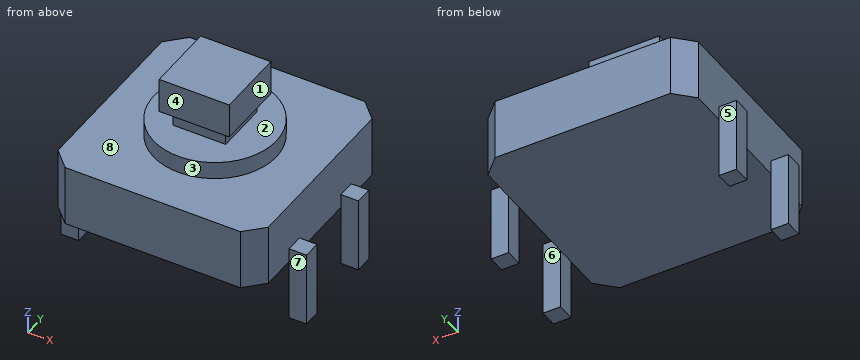
```python
from build123d import *

# Parameters (mm, degrees)
SKETCH_1_W      = 12
SKETCH_1_H      = 12
EXTRUDE_1_DEPTH = 3.5
SKETCH_2_R      = 3.5
EXTRUDE_2_DEPTH = 1
SKETCH_3_W      = 3
SKETCH_3_H      = 3
EXTRUDE_3_DEPTH = 1
SKETCH_4_W      = 4
SKETCH_4_H      = 4
EXTRUDE_4_DEPTH = 2
SKETCH_5_W      = 4.3
SKETCH_5_H      = 1
EXTRUDE_5_DEPTH = 1
SKETCH_7_W      = 4.3
SKETCH_7_H      = 1
EXTRUDE_6_DEPTH = 1
CHAMFER_1_SIZE  = 1


with BuildPart() as part:
    # 스케치1 → 보스-돌출1 (new body)
    with BuildSketch(Plane.XY):
        Rectangle(SKETCH_1_W, SKETCH_1_H)
    extrude(amount=EXTRUDE_1_DEPTH)

    # 스케치2 → 보스-돌출2 (add)
    with BuildSketch(Plane.XY.offset(3.5)):
        Circle(SKETCH_2_R)
    extrude(amount=EXTRUDE_2_DEPTH)

    # 스케치3 → 보스-돌출3 (add)
    with BuildSketch(Plane.XY.offset(4.5)):
        Rectangle(SKETCH_3_W, SKETCH_3_H)
    extrude(amount=EXTRUDE_3_DEPTH)

    # 스케치4 → 보스-돌출4 (add)
    with BuildSketch(Plane.XY.offset(5.5)):
        Rectangle(SKETCH_4_W, SKETCH_4_H)
    extrude(amount=EXTRUDE_4_DEPTH)

    # 스케치5 → 보스-돌출5 (add)
    with BuildSketch(Plane.ZY.offset(6)):
        with Locations((-1.35, 2.5)):
            Rectangle(SKETCH_5_W, SKETCH_5_H)
        with Locations((-1.35, -2.5)):
            Rectangle(SKETCH_5_W, SKETCH_5_H)
    extrude(amount=EXTRUDE_5_DEPTH)

    # 스케치7 → 보스-돌출6 (add)
    with BuildSketch(Plane(origin=(6, 0, 0), x_dir=(0, 0, -1), z_dir=(1, 0, 0))):
        with Locations((1.35, 2.5)):
            Rectangle(SKETCH_7_W, SKETCH_7_H)
        with Locations((1.35, -2.5)):
            Rectangle(SKETCH_7_W, SKETCH_7_H)
    extrude(amount=EXTRUDE_6_DEPTH)

    # 모따기1
    chamfer_1_edges = [part.edges().sort_by_distance(p)[0] for p in [
        (6, -6, 1.75),
        (-6, -6, 1.75),
        (-6, 6, 1.75),
        (6, 6, 1.75),
    ]]
    chamfer(chamfer_1_edges, length=CHAMFER_1_SIZE)


solid = part.part
```
The model under review builds one solid part; all positions refer to its coordinate system, in mm. Face numbers are marked on the shaded views. A direction names the side the tool comes from. Give positions to 0.01 mm unless a question says otherwise; leave off trailing zeros. Order: outer loops, then holes, each group sorted by start corner. A loop starts at its lowest first (then second) coordinate and runs counter-clockwise, first axis right, second up. Notation, with made-up numbers: (27, 47) - (54, 47) arc R21 ccw to (54, 69) - close; hole circle Ø7 at (-11.5, 6). An arc over 180 degrees is marked (long way). Use CSV: the item, a comma, the result in double quotes. Start each with the question number.
Q1. We need section C-C, the plane x = 0. Write out the cut boundary in (y, z), and give its area (3 significant figures).
Q2. Tool access review of the marked faces 1, 2, 3, 4 and 5: name each direction out of +Z, -Z, +X, -X, +Y, -Y from which nothing blocks a thin tool from reaching the whole face with its end or side.
Q3. To check wall thickness, follow line 1 along X through (y, z) = (-2.25, -1); line 2 along Z through (x, y) = (-1.5, -1.75); line 3 along X through (y, z) = (3.5, 0.5). State the ranges of each line that lie inside material, in increasing order. Write a range as [from, to].
Q4. The part is to be moulded in two halves that separate along Y. For the marked faces 6, 7 and 8, say which applies: +Y half, -Y half, draft (parallel to the pull), parting line (faces both ways), or undercut.
Q5. We need section A-A, the plane z = -2.5. Write out the cut boundary in (x, y).
Q6. Clearance check with flat-ended pins moving along their axes: pin 1 Ø1 at (x, y) = (-0.5, 3.5) entering from +Z; pin 2 Ø1 at (y, z) = (-4, -1.5) entering from -X; pin 3 Ø0.6 at (x, z) = (-0.5, 6.5) entering from +Y; pin 4 Ø4 at (y, z) = (-2.5, 3) entering from +X. State where each tip first meets the part, or that it passes through.
Q7. We need section D-D, the plane z = 2.5. Write out the cut boundary in (x, y), and give its area (3 significant figures).
Outcome:
1,outline,"(-6, 0) - (6, 0) - (6, 3.5) - (3.5, 3.5) - (3.5, 4.5) - (1.5, 4.5) - (1.5, 5.5) - (2, 5.5) - (2, 7.5) - (-2, 7.5) - (-2, 5.5) - (-1.5, 5.5) - (-1.5, 4.5) - (-3.5, 4.5) - (-3.5, 3.5) - (-6, 3.5) - close"
1,area,"60.0 mm^2"
2,face 1,"+Z, +X, +Y, -Y"
2,face 2,"none"
2,face 3,"+Z"
2,face 4,"+Z, +X, -X, -Y"
2,face 5,"+Z, -Z, -X, +Y"
3,line 1,"x = [-7, -6], [6, 7]"
3,line 2,"z = [0, 4.5], [5.5, 7.5]"
3,line 3,"x = [-6, 6]"
4,face 6,"undercut"
4,face 7,"-Y half"
4,face 8,"draft"
5,outline,"(-7, -3) - (-6, -3) - (-6, -2) - (-7, -2) - close; (-7, 2) - (-6, 2) - (-6, 3) - (-7, 3) - close; (6, -3) - (7, -3) - (7, -2) - (6, -2) - close; (6, 2) - (7, 2) - (7, 3) - (6, 3) - close"
6,pin 1,"stops at z = 4.5"
6,pin 2,"passes through"
6,pin 3,"stops at y = 2"
6,pin 4,"stops at x = 6"
7,outline,"(-6, -5) - (-5, -6) - (5, -6) - (6, -5) - (6, 5) - (5, 6) - (-5, 6) - (-6, 5) - close"
7,area,"142 mm^2"
